Answer from the drawing. Dimensions are ordinates in mm from the lowest x, y and z of the part. Give positions to 0.01 mm unless a question says otherwise; leave off trailing zeros. Write each loop counter-clockwise with the first axis right and the second up, starting at its lowest first coordinate (ties: lowest second). Pieces come first, ordered by that corner, then holes. Notation, with made-up numbers: M -18.75,14 L 15.25,14 A11 ccw 15.25,23 Z; hole C 13.5,48 d7. An arc over 180 degrees is marked long. Answer as a JSON object with one key per item and string values.
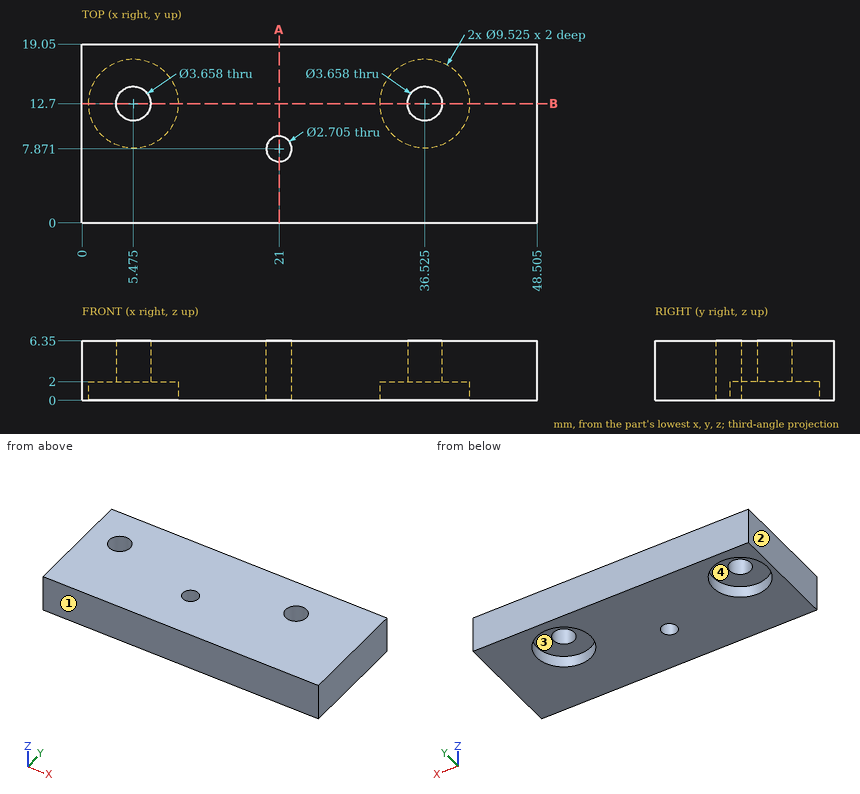
1. A cutting plane is placed at A-A, the plane x = 21. Give the vertices of the cut face in (y, z).
Verdict:
{"outline": "M 0,0 L 6.52,0 L 6.52,6.35 L 0,6.35 Z; M 9.22,0 L 19.05,0 L 19.05,6.35 L 9.22,6.35 Z"}
2. The mould has two halves that part along X. Classify the marked faces 1, 2, 3 and 4: released by +X, released by -X, zero draft, split by the parting line, or undercut.
Verdict:
{"face 1": "zero draft", "face 2": "released by -X", "face 3": "undercut", "face 4": "undercut"}
3. Consider line 1 along Y through (x, z) = (21, 4.25); line 2 along X through (y, z) = (13.5, 3.75) (1 decimal); line 3 along X through (y, z) = (14, 1.75) (1 decimal). Determine where each line is inside the solid, lowest interval first.
Verdict:
{"line 1": "y = 0 to 6.52, 9.22 to 19.05", "line 2": "x = 0 to 3.8, 7.1 to 34.9, 38.2 to 48.5", "line 3": "x = 0 to 0.9, 10.1 to 31.9, 41.1 to 48.5"}
4. Flat-ended cylindrical pins translate along their axes: pin 1 (3.5 mm diameter, centred on x = 36.525, y = 12.7, fed in from -Z); pin 2 (5.5 mm diameter, centred on x = 36.525, y = 12.7, fed in from -Z). Find the tip coordinate at first contact, or state that the pin passes through.
Verdict:
{"pin 1": "passes through", "pin 2": "stops at z = 2"}
5. A cutting plane is placed at B-B, the plane y = 12.7. Count the separate pieces of the cut face and the enclosed holes in it, plus the area to 3 significant figures.
Verdict:
{"separate pieces": "3", "enclosed holes": "0", "area": "238 mm2"}
